Read the model definition and answer for the solid it produces. Units are mm, in the model's axes. Coordinates: 2 decimals unless noted, no trailing zeros. Order: outer loops, then holes, each group sorted by start corner. A loop starts at its lowest first (then second) coordinate and runs counter-clockwise, first axis right, second up.
from build123d import *

# Parameters (mm, degrees)
BOSS_EXTRUDE1_DEPTH = 4
SKETCH2_R           = 1.5
CUT_EXTRUDE1_DEPTH  = 4
CIRPATTERN1_COUNT   = 3
SKETCH3_R           = 10.25
CUT_EXTRUDE2_DEPTH  = 4
SKETCH4_R           = 2
CUT_EXTRUDE3_DEPTH  = 4
CIRPATTERN2_COUNT   = 2
CIRPATTERN2_ANGLE   = 90


with BuildPart() as part:
    # Sketch1 → Boss-Extrude1 (new body)
    with BuildSketch(Plane(origin=(0, 0, 0), x_dir=(1, 0, 0), z_dir=(0, 1, 0))):
        with BuildLine():
            ThreePointArc((-30, 0), (0, 30), (30, 0))
            ThreePointArc((30, 0), (0, -30), (-30, 0))
        make_face()
    extrude(amount=BOSS_EXTRUDE1_DEPTH)

    # Sketch2 → Cut-Extrude1 (cut)
    with BuildSketch(Plane(origin=(0, 4, 0), x_dir=(1, 0, 0), z_dir=(0, 1, 0))):
        with Locations(Location((7.5, 12.990381057, 0), (0, 0, 270))):
            Circle(SKETCH2_R)
    cut_extrude1 = extrude(amount=-CUT_EXTRUDE1_DEPTH, mode=Mode.SUBTRACT)

    # CirPattern1: Cut-Extrude1 ×3 about axis
    cirpattern1_axis = Axis((0, 0, 0), (0, 1, 0))
    for i in range(1, CIRPATTERN1_COUNT):
        add(cut_extrude1.rotate(cirpattern1_axis, i * 360 / CIRPATTERN1_COUNT), mode=Mode.SUBTRACT)

    # Sketch3 → Cut-Extrude2 (cut)
    with BuildSketch(Plane(origin=(0, 4, 0), x_dir=(1, 0, 0), z_dir=(0, 1, 0))):
        with Locations(Location((0, 0, 0), (0, 0, 270))):
            Circle(SKETCH3_R)
    extrude(amount=-CUT_EXTRUDE2_DEPTH, mode=Mode.SUBTRACT)

    # Sketch4 → Cut-Extrude3 (cut)
    with BuildSketch(Plane(origin=(0, 4, 0), x_dir=(1, 0, 0), z_dir=(0, 1, 0))):
        with Locations(Location((6.59989, -24.631107405, 0), (0, 0, 270))):
            Circle(SKETCH4_R)
    cut_extrude3 = extrude(amount=-CUT_EXTRUDE3_DEPTH, mode=Mode.SUBTRACT)

    # CirPattern2: Cut-Extrude3 ×2 about axis
    cirpattern2_axis = Axis((0, 4, 0), (0, 1, 0))
    for i in range(1, CIRPATTERN2_COUNT):
        add(cut_extrude3.rotate(cirpattern2_axis, i * CIRPATTERN2_ANGLE / (CIRPATTERN2_COUNT - 1)), mode=Mode.SUBTRACT)


solid = part.part
Q1. The part is cut by section C-C, the plane y = 3.35. Determine the outline of the cut face in (x, z).
Q2. The part is cut by section D-D, the plane x = 7.5. Determine the outline of the cut face in (y, z), then the cut area to 3 significant figures.
Q3. Straight lines are drawn through the part: L1, parallel to X at y = 1.3, z = 9; L2, parallel to X at y = 1.05, z = -6.5; L3, parallel to Z at x = -15, y = 3.2. For each, find the intervals that lie inside material, in ascending order.
Q4. The part is cut by section B-B, the plane x = 0. Determine the outline of the cut face in (y, z), then the cut area to 3 significant figures.
Q5. Determine the mould class of faces 1 (the cylindrical face through (-6.503, 1.972, -29.287)), 2 (the cylindrical face through (6.587, 2.028, -14.181)), 3 (the flat face through (-13, 0, 0)) for opening direction Z: +Z half, -Z half, draft (parallel to the pull), parting line (faces both ways), or undercut.
Q6. The part is cut by section A-A, the plane z = 0. Determine the outline of the cut face in (x, y), then the cut area to 3 significant figures.
Computed values:
1. outline: circle Ø60 at (0, 0); hole circle Ø3 at (-15, 0); hole circle Ø20.5 at (0, 0); hole circle Ø4 at (6.6, 24.63); hole circle Ø3 at (7.5, -12.99); hole circle Ø3 at (7.5, 12.99); hole circle Ø4 at (24.63, -6.6)
2. outline: (0, -29.05) - (4, -29.05) - (4, -14.49) - (0, -14.49) - close; (0, -11.49) - (4, -11.49) - (4, -6.99) - (0, -6.99) - close; (0, 6.99) - (4, 6.99) - (4, 11.49) - (0, 11.49) - close; (0, 14.49) - (4, 14.49) - (4, 22.85) - (0, 22.85) - close; (0, 26.42) - (4, 26.42) - (4, 29.05) - (0, 29.05) - close
2. area: 138 mm2
3. L1: x = -28.62 to -4.91, 4.91 to 28.62
3. L2: x = -29.29 to -7.93, 7.93 to 22.63, 26.63 to 29.29
3. L3: z = -25.98 to -1.5, 1.5 to 25.98
4. outline: (0, -30) - (4, -30) - (4, -10.25) - (0, -10.25) - close; (0, 10.25) - (4, 10.25) - (4, 30) - (0, 30) - close
4. area: 158 mm2
5. face 1: parting line
5. face 2: undercut
5. face 3: draft
6. outline: (-30, 0) - (-16.5, 0) - (-16.5, 4) - (-30, 4) - close; (-13.5, 0) - (-10.25, 0) - (-10.25, 4) - (-13.5, 4) - close; (10.25, 0) - (30, 0) - (30, 4) - (10.25, 4) - close
6. area: 146 mm2
